Drawing for the job (mm, zero at the part's lowest x, y, z). A direction names the side the tool comes from. Round coordinates to 2 decimals unless told otherwise and drop trailing zeros. Loops run counter-clockwise (first coordinate to the right, second up) from the corner with the lowest first, then second, coordinate; pieces in that order, holes last. Notation, with made-up numbers: M 41,-26.5 L 94,-26.5 A33 cw 94,2.5 Z; hole C 15.5,33 d11. An arc over 180 degrees is marked long. Answer in a Markdown table with one row per item.
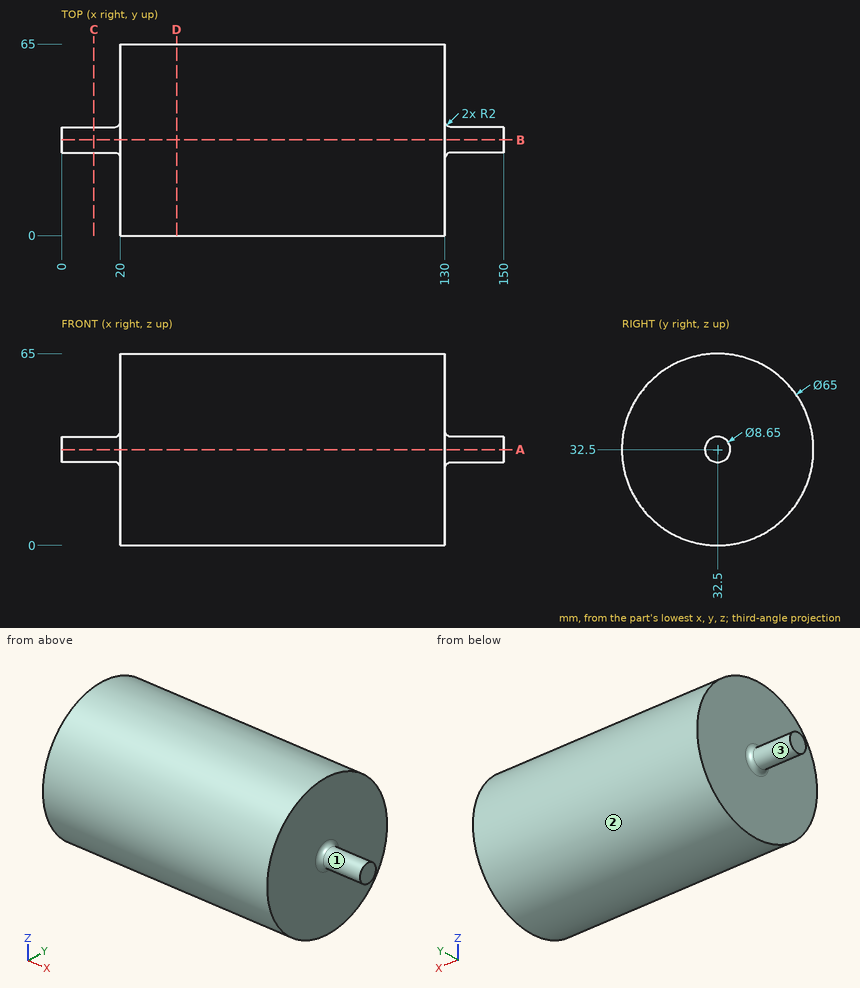
1. Saw through at D-D (x = 39). Write the cut outline in (y, z).
Verdict:
| item | result |
|---|---|
| outline | C 32.5,32.5 d65 |
2. Wall check: probe 1 along X at (y, z) = (54, 20); probe 2 along Y at (x, z) = (18, 33); probe 3 along Y at (x, z) = (106.5, 51). Give the ranges that are in metal, low to high.
Verdict:
| item | result |
|---|---|
| probe 1 | x = 20 to 130 |
| probe 2 | y = 28.2 to 36.8 |
| probe 3 | y = 5.78 to 59.22 |
3. Pin check, flat tips, straight feed: pin 1 (1.5 mm diameter, centred on x = 41.5, z = 38.5, fed in from -Y); pin 2 (8 mm diameter, centred on x = 97, y = 13.5, fed in from +Z); pin 3 (2 mm diameter, centred on y = 15.5, z = 46, fed in from -X); pin 4 (19.5 mm diameter, centred on y = 40, z = 35, fed in from -X). Stop position of each tip, or through.
Verdict:
| item | result |
|---|---|
| pin 1 | stops at y = 0.43 |
| pin 2 | stops at z = 61.33 |
| pin 3 | stops at x = 20 |
| pin 4 | stops at x = 0 |
4. Saw through at A-A (z = 32.5). Write the cut outline in (x, y) (3 decimals).
Verdict:
| item | result |
|---|---|
| outline | M 0,28.175 L 18,28.175 A2 cw 20,26.175 L 20,0 L 130,0 L 130,26.175 A2 cw 132,28.175 L 150,28.175 L 150,36.825 L 132,36.825 A2 cw 130,38.825 L 130,65 L 20,65 L 20,38.825 A2 cw 18,36.825 L 0,36.825 Z |
5. Saw through at C-C (x = 11). Write the cut outline in (y, z) (3 decimals), and give its area (3 significant figures).
Verdict:
| item | result |
|---|---|
| outline | C 32.5,32.5 d8.65 |
| area | 58.8 mm² |
6. Tool access for the marked faces 1, 2 and 3: list every direction of +Z, -Z, +X, -X, +Y, -Y with a clear straight run to the whole face (end or side of a thin tool).
Verdict:
| item | result |
|---|---|
| face 1 | +X |
| face 2 | +X, -X |
| face 3 | -X |
